Read the model definition and answer for the solid it produces. Units are mm, in the model's axes. Face numbers are marked on the shaded views. A direction names the side the tool comes from. Coordinates: 2 decimals unless noted, no trailing zeros. Write each loop counter-clockwise with the first axis right and the second up, starting at its lowest first coordinate (ties: lowest second). Pieces come first, ordered by that corner, then holes.
Item 1: A tool of negligible diameter and unlimited length cuts with its end or side. For the marked faces 1 and 2, from which of +Z, -Z, +X, -X, +Y, -Y can it reach the whole face along a straight path? Write none if from no direction.
Item 2: Section C-C (y = 13.75) is taken. Give the vertices of the cut face in (x, z), then the cut area to 3 significant figures.
Item 3: Section B-B (z = 0) is taken. Give the vertices of the cut face in (x, y), then the cut area to 3 significant figures.
Item 4: Each of these flat-tipped pins is pushed along its axis until it touches: P1, Ø1, axis at x = 1, y = 1.5, coming from the +Z side; P2, Ø0.6, axis at x = -2, z = 0, coming from the -Y side. Where does it stop, or does it pass through?
Item 5: Section D-D (y = 3.25) is taken. Give the vertices of the cut face in (x, z).
Item 6: Straight lines are drawn through the part: probe 1 along X at (y, z) = (0.15, 0); probe 2 along Y at (x, z) = (1.5, 1); probe 3 along Z at (x, y) = (-2.5, 1.25). For each, find the intervals that lie inside material, in ascending order.
Item 7: Section A-A (x = 0) is taken. Give the vertices of the cut face in (y, z), then the cut area to 3 significant figures.
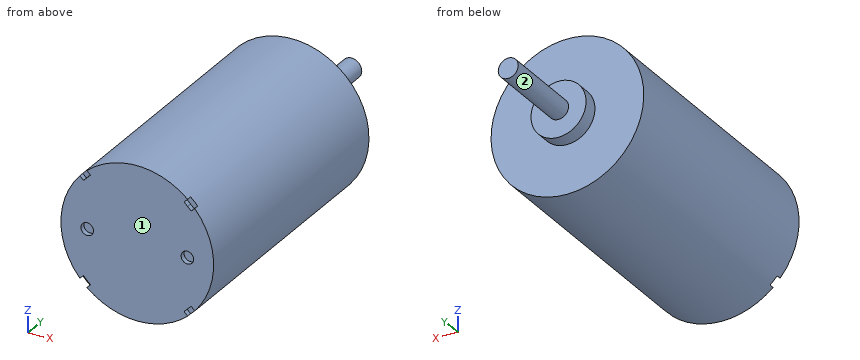
from build123d import *

# Parameters (mm, degrees)
SKETCH_1_W               = 0.4
SKETCH_1_H               = 3.4
SKETCH_1_W_2             = 3.05
SKETCH_1_H_2             = 10.5
CUT_EXTRUDE_START        = -0.2
CUT_EXTRUDE_1_DEPTH      = 0.2
PATTERN_CIRCULAR_1_COUNT = 4
SKETCH_2_3_R             = 0.25
CUT_EXTRUDE_2_DEPTH      = 0.2


with BuildPart() as part:
    # Sketch 1 → Revolve 1 (revolve)
    with BuildSketch(Plane(origin=(0, 0, 0), x_dir=(0, 0, -1), z_dir=(1, 0, 0))):
        with Locations((0.2, 12.8)):
            Rectangle(SKETCH_1_W, SKETCH_1_H)
        Polygon((0, 11.1), (0, 10.5), (1.1, 10.5), (1.1, 11.1), (0.4, 11.1), align=None)
        with Locations((1.525, 5.25)):
            Rectangle(SKETCH_1_W_2, SKETCH_1_H_2)
    revolve(axis=Axis((0, 11.1, 0), (0, 1, 0)))

    # Sketch 2 → Cut-Extrude 1 (cut)
    with BuildSketch(Plane.XZ.offset(CUT_EXTRUDE_START)):
        with BuildLine():
            Line((-2.152033922, 1.869191209), (-2.010612565, 2.010612565))
            Line((-2.010612565, 2.010612565), (-1.869191209, 2.152033922))
            Line((-1.869191209, 2.152033922), (-2.010612565, 2.293455278))
            ThreePointArc((-2.010612565, 2.293455278), (-2.156675683, 2.156675683), (-2.293455278, 2.010612565))
            Line((-2.293455278, 2.010612565), (-2.152033922, 1.869191209))
        make_face()
    cut_extrude_1 = extrude(amount=CUT_EXTRUDE_1_DEPTH, mode=Mode.SUBTRACT)

    # Pattern Circular 1: Cut-Extrude 1 ×4 about axis
    pattern_circular_1_axis = Axis((0, 0, 0), (0, 1, 0))
    for i in range(1, PATTERN_CIRCULAR_1_COUNT):
        add(cut_extrude_1.rotate(pattern_circular_1_axis, i * 360 / PATTERN_CIRCULAR_1_COUNT), mode=Mode.SUBTRACT)

    # Sketch 2_3 → Cut-Extrude 2 (cut)
    with BuildSketch(Plane.XZ):
        with Locations(Location((-2, 0, 0), (0, 0, 270))):
            Circle(SKETCH_2_3_R)
        with Locations(Location((2, 0, 0), (0, 0, 270))):
            Circle(SKETCH_2_3_R)
    extrude(amount=-CUT_EXTRUDE_2_DEPTH, mode=Mode.SUBTRACT)


solid = part.part
Established:
1. face 1: +Z, -Z, +X, -X, -Y
1. face 2: +Y
2. outline: circle Ø0.8 at (0, 0)
2. area: 0.503 mm2
3. outline: (-3.05, 0) - (-2.25, 0) - (-2.25, 0.2) - (-1.75, 0.2) - (-1.75, 0) - (1.75, 0) - (1.75, 0.2) - (2.25, 0.2) - (2.25, 0) - (3.05, 0) - (3.05, 10.5) - (1.1, 10.5) - (1.1, 11.1) - (0.4, 11.1) - (0.4, 14.5) - (-0.4, 14.5) - (-0.4, 11.1) - (-1.1, 11.1) - (-1.1, 10.5) - (-3.05, 10.5) - close
3. area: 67.9 mm2
4. P1: stops at z = 3.01
4. P2: stops at y = 0
5. outline: circle Ø6.1 at (0, 0)
6. probe 1: x = -3.05 to -2.25, -1.75 to 1.75, 2.25 to 3.05
6. probe 2: y = 0 to 10.5
6. probe 3: z = -1.75 to 1.75
7. outline: (0, -3.05) - (10.5, -3.05) - (10.5, -1.1) - (11.1, -1.1) - (11.1, -0.4) - (14.5, -0.4) - (14.5, 0.4) - (11.1, 0.4) - (11.1, 1.1) - (10.5, 1.1) - (10.5, 3.05) - (0, 3.05) - close
7. area: 68.1 mm2
